Work out the finished part from the listing and answer in its coordinate system (mm). A direction names the side the tool comes from. Give positions to 0.01 mm unless a question says otherwise; leave off trailing zeros. Loops run counter-clockwise (first coordinate to the right, second up) from the corner with the lowest first, then second, coordinate; pieces in that order, holes last. Notation, with made-up numbers: (79.5, -38) - (83.5, -38) arc R13 cw to (83.5, -33) - close; hole circle Ø4 at (46.25, 37). An arc over 180 degrees is marked (long way). One line per question, with ' | ' between items. Start each with the question number.
1. Find the intervals of material crossed by line 1 (Z direction, x = -159, y = 0); line 2 (Z direction, x = -348, y = 42); line 3 (Y direction, x = -21, z = 18), in increasing order.
2. Which of the six approach directions +Z, -Z, +X, -X, +Y, -Y give full straight-line access (tool end or side, diameter ignored) to faces 1 (the face through (-162.52, 3.57, 43.92)), 2 (the face through (-156.172, -3.435, 43.917)), 3 (the face through (-278.676, -4.862, 3.219)), 4 (the face through (-365.67, 8.04, 3.13))?
3. Section B-B (x = -200) is taken. Determine the outline of the cut face in (y, z).
4. Section D-D (x = -265.5) is taken. Determine the outline of the cut face in (y, z).
5. Each of these flat-tipped pins is pushed along its axis until it touches: pin 1 (1.5 mm diameter, centred on y = -59, z = 64, fed in from +X); pin 2 (5 mm diameter, centred on y = -22, z = 50.5, fed in from -X); pin 3 (1.5 mm diameter, centred on y = 144.5, z = 33, fed in from -X); pin 4 (7.5 mm diameter, centred on y = 0, z = 38.1, fed in from +X). Where does it stop, or does it pass through?
6. Section A-A (y = -83) is taken. Determine the outline of the cut face in (x, z), plus the area to 3 significant figures.
7. For a pull along X with two mould halves and no side action, classify faces 5 (the face through (-207.898, 3.286, 3.219)), 6 (the face through (-111.733, 2.458, 3.131)), 7 (the face through (-226, 5, 6.35)) as released by +X, released by -X, zero draft, split by the parting line, or undercut.
8. Section C-C (x = -72.5) is taken. Determine the outline of the cut face in (y, z).
from build123d import *

# Parameters (mm, degrees)
F0_R     = 365.76
F0_R_2   = 111.76
F1_DEPTH = 6.35
F2_W     = 380.011261
F2_H     = 787.612766
F3_DEPTH = 6.351
F5_DEPTH = 6.351
F7_DEPTH = 76.2
F8_R     = 6.35
F9_DEPTH = 365.761


with BuildPart() as f1:
    # F0 (on Top) → F1 (new body)
    with BuildSketch(Plane.XY):
        Circle(F0_R)
        Circle(F0_R_2, mode=Mode.SUBTRACT)
    extrude(amount=F1_DEPTH)

    # F2 (on face) → F3 (cut, through all)
    with BuildSketch(Plane.XY.offset(6.35)):
        with Locations((190.00563, 1.120374)):
            Rectangle(F2_W, F2_H)
    extrude(amount=-F3_DEPTH, mode=Mode.SUBTRACT)

    # F4 (on face) → F5 (cut, through all)
    with BuildSketch(Plane.XY.offset(6.35)):
        with BuildLine():
            ThreePointArc((-88.9, 289.56), (-302.899659, 0), (-88.9, -289.56))
            Line((-88.9, -289.56), (-88.9, -264.16))
            ThreePointArc((-88.9, -264.16), (-278.717986, 0), (-88.9, 264.16))
            Line((-88.9, 264.16), (-88.9, 289.56))
        make_face()
        with BuildLine():
            ThreePointArc((-88.9, 187.96), (-207.923475, 0), (-88.9, -187.96))
            Line((-88.9, -187.96), (-88.9, -162.56))
            ThreePointArc((-88.9, -162.56), (-185.28077, 0), (-88.9, 162.56))
            Line((-88.9, 162.56), (-88.9, 187.96))
        make_face()
    extrude(amount=-F5_DEPTH, mode=Mode.SUBTRACT)

    # F6 (on face) → F7 (join)
    with BuildSketch(Plane.XY.offset(6.35)):
        with BuildLine():
            Line((0, 156.21), (0, 162.56))
            ThreePointArc((0, 162.56), (-162.56, 0), (0, -162.56))
            Line((0, -162.56), (0, -156.21))
            ThreePointArc((0, -156.21), (-156.21, 0), (0, 156.21))
        make_face()
    extrude(amount=F7_DEPTH)

    # F8 (on Right) → F9 (cut, through all)
    with BuildSketch(Plane.YZ):
        with Locations((0, 38.1)):
            Circle(F8_R)
    extrude(amount=-F9_DEPTH, mode=Mode.SUBTRACT)


solid = f1.part
Conclusion:
1) line 1: 0 to 31.75, 44.45 to 82.55 | line 2: 0 to 6.35 | line 3: -161.2 to -154.79, 154.79 to 161.2
2) face 1: +Z, -X | face 2: +Z, +X | face 3: +Z, -Z | face 4: +Z, -Z, -X
3) outline: (-306.24, 0) - (-227.48, 0) - (-227.48, 6.35) - (-306.24, 6.35) - close; (-194.12, 0) - (-56.85, 0) - (-56.85, 6.35) - (-194.12, 6.35) - close; (56.85, 0) - (194.12, 0) - (194.12, 6.35) - (56.85, 6.35) - close; (227.48, 0) - (306.24, 0) - (306.24, 6.35) - (227.48, 6.35) - close
4) outline: (-251.58, 0) - (-145.8, 0) - (-145.8, 6.35) - (-251.58, 6.35) - close; (-84.81, 0) - (84.81, 0) - (84.81, 6.35) - (-84.81, 6.35) - close; (145.8, 0) - (251.58, 0) - (251.58, 6.35) - (145.8, 6.35) - close
5) pin 1: x = -144.33 | pin 2: x = -161.39 | pin 3: x = -75.91 | pin 4: through
6) outline: (-356.22, 0) - (-291.31, 0) - (-291.31, 6.35) - (-356.22, 6.35) - close; (-266.07, 0) - (-190.64, 0) - (-190.64, 6.35) - (-266.07, 6.35) - close; (-165.65, 0) - (-74.84, 0) - (-74.84, 6.35) - (-132.34, 6.35) - (-132.34, 82.55) - (-139.77, 82.55) - (-139.77, 6.35) - (-165.65, 6.35) - close | area: 2,030 mm²
7) face 5: undercut | face 6: released by +X | face 7: zero draft
8) outline: (-358.5, 0) - (-85.05, 0) - (-85.05, 6.35) - (-138.37, 6.35) - (-138.37, 82.55) - (-145.5, 82.55) - (-145.5, 6.35) - (-358.5, 6.35) - close; (85.05, 0) - (358.5, 0) - (358.5, 6.35) - (145.5, 6.35) - (145.5, 82.55) - (138.37, 82.55) - (138.37, 6.35) - (85.05, 6.35) - close
